Could you check a few things on this model? Use its own coordinates, in mm. Coordinates: 2 decimals unless noted, no trailing zeros. Loops run counter-clockwise (first coordinate to the right, second up) from the corner with the lowest first, then second, coordinate; pieces in that order, holes last.
Autodesk Inventor part; units mm, degrees
ref_plane "YZ Plane" through (0, 0, 0) normal (1, 0, 0) x (0, 1, 0)
ref_plane "XZ Plane" through (0, 0, 0) normal (0, 1, 0) x (-1, 0, 0)
ref_plane "XY Plane" through (0, 0, 0) normal (0, 0, 1) x (1, 0, 0)
sketch "Sketch1" plane through (0, 0, 0) normal (0, 0, 1) x (1, 0, 0)
  circle A0 centre (0, 0) radius 18.5
  circle A1 centre (0, 0) radius 14.5
  dimension "d0" = 37
  dimension "d1" = 29
extrude "Extrusion1" add sketch "Sketch1" along normal blind 6.2
thread "Thread1"
chamfer "Chamfer1" distance 1 angle 45 2 edges at (-14.5, 0, 6.2) (-14.5, 0, 0)
fillet "Fillet1" radius 0.5 2 edges at (-18.5, 0, 6.2) (-18.5, 0, 0)
properties part number "13536_Ring"
(1) For pin 1 (10 mm diameter, centred on x = -1, y = 9.5, fed in from -Z); pin 2 (4 mm diameter, centred on x = -1, y = 12.5, fed in from -Z); pin 3 (3 mm diameter, centred on x = 6.5, z = 2.5, fed in from -Y), each with a flat end and sliding along its axis, tell me the tip position at first contact or that it passes through.
Answers:
pin 1: stops at z = 0.95
pin 2: stops at z = 0.96
pin 3: stops at y = -17.81
(2) Imagine slicing it at C-C, the plane z = 2.75. Write out the boundary of the cut face in (x, y), and give its area (3 significant figures).
Answers:
outline: circle Ø37 at (0, 0); hole circle Ø29 at (0, 0)
area: 415 mm2
(3) Imagine slicing it at A-A, the plane y = 0. Write out the boundary of the cut face in (x, z).
Answers:
outline: (-18.5, 0.5) arc R0.5 ccw to (-18, 0) - (-15.5, 0) - (-14.5, 1) - (-14.5, 5.2) - (-15.5, 6.2) - (-18, 6.2) arc R0.5 ccw to (-18.5, 5.7) - close; (14.5, 1) - (15.5, 0) - (18, 0) arc R0.5 ccw to (18.5, 0.5) - (18.5, 5.7) arc R0.5 ccw to (18, 6.2) - (15.5, 6.2) - (14.5, 5.2) - close
(4) I need wall thicknesses on probe 1 along Y at (x, z) = (0, 2.7); probe 2 along Y at (x, z) = (-13, 0.75); probe 3 along X at (y, z) = (1, 0.5). Which ranges of each line are inside material? Lowest first, please.
Answers:
probe 1: y = -18.5 to -14.5, 14.5 to 18.5
probe 2: y = -13.16 to -6.97, 6.97 to 13.16
probe 3: x = -18.47 to -14.97, 14.97 to 18.47
(5) We'd pull the mould along X, two halves only. Please class faces 1 (the face through (-4.01, 18.06, 3.06)), 2 (the face through (6.691, 12.864, 3.071)), 3 (the face through (5, 15, 6.2)): +X half, -X half, draft (parallel to the pull), parting line (faces both ways), or undercut.
Answers:
face 1: parting line
face 2: undercut
face 3: draft
